```python
from build123d import *

# Parameters (mm, degrees)
SKETCH1_R           = 25
BOSS_EXTRUDE1_DEPTH = 10
SKETCH2_R           = 34
SKETCH2_R_2         = 1.27
BOSS_EXTRUDE2_DEPTH = 10
SKETCH3_R           = 3
CUT_EXTRUDE1_DEPTH  = 53.076866265
CUT_EXTRUDE2_DEPTH  = 2.5


with BuildPart() as part:
    # Sketch1 → Boss-Extrude1 (new body)
    with BuildSketch(Plane(origin=(0, 0, 0), x_dir=(1, 0, 0), z_dir=(0, 1, 0))):
        with Locations(Location((0, 0, 0), (0, 0, 270))):
            Circle(SKETCH1_R)
        with BuildLine():
            Line((-1.5, 11), (1.5, 11))
            Line((1.5, 11), (2.425924848, 8.146464793))
            ThreePointArc((2.425924848, 8.146464793), (3.252809175, 7.852976026), (4.045032587, 7.475808409))
            Line((4.045032587, 7.475808409), (6.717514421, 8.838834765))
            Line((6.717514421, 8.838834765), (8.838834765, 6.717514421))
            Line((8.838834765, 6.717514421), (7.475808409, 4.045032587))
            ThreePointArc((7.475808409, 4.045032587), (7.852976026, 3.252809175), (8.146464793, 2.425924848))
            Line((8.146464793, 2.425924848), (11, 1.5))
            Line((11, 1.5), (11, -1.5))
            Line((11, -1.5), (8.146464793, -2.425924848))
            ThreePointArc((8.146464793, -2.425924848), (7.852976026, -3.252809175), (7.475808409, -4.045032587))
            Line((7.475808409, -4.045032587), (8.838834765, -6.717514421))
            Line((8.838834765, -6.717514421), (6.717514421, -8.838834765))
            Line((6.717514421, -8.838834765), (4.045032587, -7.475808409))
            ThreePointArc((4.045032587, -7.475808409), (3.252809175, -7.852976026), (2.425924848, -8.146464793))
            Line((2.425924848, -8.146464793), (1.5, -11))
            Line((1.5, -11), (-1.5, -11))
            Line((-1.5, -11), (-2.425924848, -8.146464793))
            ThreePointArc((-2.425924848, -8.146464793), (-3.252809175, -7.852976026), (-4.045032587, -7.475808409))
            Line((-4.045032587, -7.475808409), (-6.717514421, -8.838834765))
            Line((-6.717514421, -8.838834765), (-8.838834765, -6.717514421))
            Line((-8.838834765, -6.717514421), (-7.475808409, -4.045032587))
            ThreePointArc((-7.475808409, -4.045032587), (-7.852976026, -3.252809175), (-8.146464793, -2.425924848))
            Line((-8.146464793, -2.425924848), (-11, -1.5))
            Line((-11, -1.5), (-11, 1.5))
            Line((-11, 1.5), (-8.146464793, 2.425924848))
            ThreePointArc((-8.146464793, 2.425924848), (-7.852976026, 3.252809175), (-7.475808409, 4.045032587))
            Line((-7.475808409, 4.045032587), (-8.838834765, 6.717514421))
            Line((-8.838834765, 6.717514421), (-6.717514421, 8.838834765))
            Line((-6.717514421, 8.838834765), (-4.045032587, 7.475808409))
            ThreePointArc((-4.045032587, 7.475808409), (-3.252809175, 7.852976026), (-2.425924848, 8.146464793))
            Line((-2.425924848, 8.146464793), (-1.5, 11))
        make_face(mode=Mode.SUBTRACT)
    extrude(amount=BOSS_EXTRUDE1_DEPTH)

    # Sketch2 → Boss-Extrude2 (add)
    with BuildSketch(Plane(origin=(0, 10, 0), x_dir=(1, 0, 0), z_dir=(0, 1, 0))):
        with Locations(Location((0, 0, 0), (0, 0, 270))):
            Circle(SKETCH2_R)
        with Locations(Location((0, 0, 0), (0, 0, 270))):
            Circle(SKETCH2_R_2, mode=Mode.SUBTRACT)
    extrude(amount=BOSS_EXTRUDE2_DEPTH)

    # Sketch3 → Cut-Extrude1 (cut, through all)
    with BuildSketch(Plane(origin=(0, 20, 0), x_dir=(1, 0, 0), z_dir=(0, 1, 0))):
        with Locations(Location((-5, 0, 0), (0, 0, 270))):
            Circle(SKETCH3_R)
    extrude(amount=-CUT_EXTRUDE1_DEPTH, mode=Mode.SUBTRACT)

    # Sketch4 → Cut-Extrude2 (cut)
    with BuildSketch(Plane(origin=(0, 0, 0), x_dir=(-1, 0, 0), z_dir=(0, -1, 0))):
        Polygon((-20.068660666, 1.384852309), (-19.421525249, 1.384852309), (-19.421525249, -2.115147691), (-19.735627813, -2.115147691), (-19.735627813, 1.02587795), (-20.274089352, 1.02587795), align=None)
        Polygon((-17.895884224, 1.384852309), (-15.74203807, 1.384852309), (-17.581781659, -2.20489128), (-17.853115794, -2.055552338), (-16.27348839, 1.02587795), (-17.895884224, 1.02587795), align=None)
    extrude(amount=-CUT_EXTRUDE2_DEPTH, mode=Mode.SUBTRACT)


solid = part.part
```
Read the model definition and answer for the solid it produces. Units are mm, in the model's axes. A direction names the side the tool comes from. Round coordinates to 2 decimals unless told otherwise and drop trailing zeros. Loops run counter-clockwise (first coordinate to the right, second up) from the corner with the lowest first, then second, coordinate; pieces in that order, holes last. Notation, with made-up numbers: (74.5, 46) -> (114.5, 46) arc R26 ccw to (114.5, 77) -> close; hole circle Ø8 at (23.5, -35). An arc over 180 degrees is marked (long way). One line per item, written item: value.
1) For faces 5 (the face through (3, 10, 0)), 6 (the face through (-7.662, 15.07, 1.384)), determine the directions among +Z, -Z, +X, -X, +Y, -Y from which every point of the face is accessible in a straight line to the end or side of a thin tool.
Answer list:
face 5: -Y
face 6: +Y, -Y
2) Flat-ended cylindrical pins translate along their axes: P1, Ø6.5, axis at x = -2, z = 3, coming from the -Y side; P2, Ø2.5, axis at x = 17.5, y = 1.5, coming from the +Z side; P3, Ø6, axis at x = -17.5, y = 8, coming from the -Z side. Find the tip coordinate at first contact, or state that the pin passes through.
Answer list:
P1: stops at y = 10
P2: stops at z = 19
P3: stops at z = -30.38
3) The mould has two halves that part along X. Classify faces 1 (the face through (18, 10, -18)), 2 (the face through (7.509, 4.93, 23.846)), 3 (the face through (-3.26, 4.93, -7.85)), 4 (the face through (1.26, 14.93, -0.17)): pulls with the +X half, pulls with the -X half, needs draft (parallel to the pull), parting line crosses it, or undercut.
Answer list:
face 1: needs draft
face 2: parting line crosses it
face 3: undercut
face 4: undercut
4) A cutting plane is placed at D-D (z = 23.5). Determine the outline of the cut face in (x, y).
Answer list:
outline: (-24.57, 10) -> (-8.53, 10) -> (-8.53, 0) -> (8.53, 0) -> (8.53, 10) -> (24.57, 10) -> (24.57, 20) -> (-24.57, 20) -> close
5) A cutting plane is placed at A-A (x = 0). Determine the outline of the cut face in (y, z).
Answer list:
outline: (0, -25) -> (10, -25) -> (10, -34) -> (20, -34) -> (20, -1.27) -> (10, -1.27) -> (10, -11) -> (0, -11) -> close; (0, 11) -> (10, 11) -> (10, 1.27) -> (20, 1.27) -> (20, 34) -> (10, 34) -> (10, 25) -> (0, 25) -> close
6) A cutting plane is placed at C-C (z = 0). Determine the outline of the cut face in (x, y).
Answer list:
outline: (-34, 10) -> (-25, 10) -> (-25, 0) -> (-11, 0) -> (-11, 10) -> (-8, 10) -> (-8, 20) -> (-34, 20) -> close; (-2, 10) -> (-1.27, 10) -> (-1.27, 20) -> (-2, 20) -> close; (1.27, 10) -> (11, 10) -> (11, 0) -> (16.45, 0) -> (16.45, 2.5) -> (16.8, 2.5) -> (16.8, 0) -> (19.42, 0) -> (19.42, 2.5) -> (19.74, 2.5) -> (19.74, 0) -> (25, 0) -> (25, 10) -> (34, 10) -> (34, 20) -> (1.27, 20) -> close
7) Consider L1, parallel to X at y = 14, z = 0; L2, parallel to X at y = 17, z = 0.5; L3, parallel to Y at x = -28.5, z = -10. Determine where each line is inside the solid, lowest interval first. Write a range as [from, to].
Answer list:
L1: x = [-34, -8], [-2, -1.27], [1.27, 34]
L2: x = [-34, -7.96], [-2.04, -1.17], [1.17, 34]
L3: y = [10, 20]
